For this review, use the dimensioned drawing (mm, ordinates from the lowest corner) and the shaded views. Coordinates: 2 decimals unless noted, no trailing zeros. Loops run counter-clockwise (first coordinate to the right, second up) from the corner with the lowest first, then second, coordinate; pieces in that order, holes last.
1. Take a section at B-B, the plane z = 15. State the section outline as (x, y) points, then the cut area to 3 significant figures.
2. Take a section at C-C, the plane x = 53.5. State the section outline as (y, z) points.
3. Mouldability with a two-part tool opening along Y and no side actions: class the marked faces 1 and 2 as pulls with the +Y half, pulls with the -Y half, needs draft (parallel to the pull), parting line crosses it, or undercut.
4. Take a section at D-D, the plane y = 12. State the section outline as (x, z) points.
5. Take a section at A-A, the plane y = 22.5. State the section outline as (x, z) points, then the cut area to 4 significant figures.
6. Clearance check with flat-ended pins moving along their axes: P1, Ø22.5, axis at x = 80.5, y = 12, coming from the +Z side; P2, Ø11, axis at y = 22.5, z = 14.5, coming from the -X side; P3, Ø5.5, axis at x = 53, z = 13, coming from the -Y side. State where each tip first meets the part, or that it passes through.
7. To check wall thickness, follow probe 1 along Y at (x, z) = (114.7, 2); probe 2 along X at (y, z) = (27, 4.25); probe 3 along X at (y, z) = (42.7, 4). State the ranges of each line that lie inside material, in increasing order.
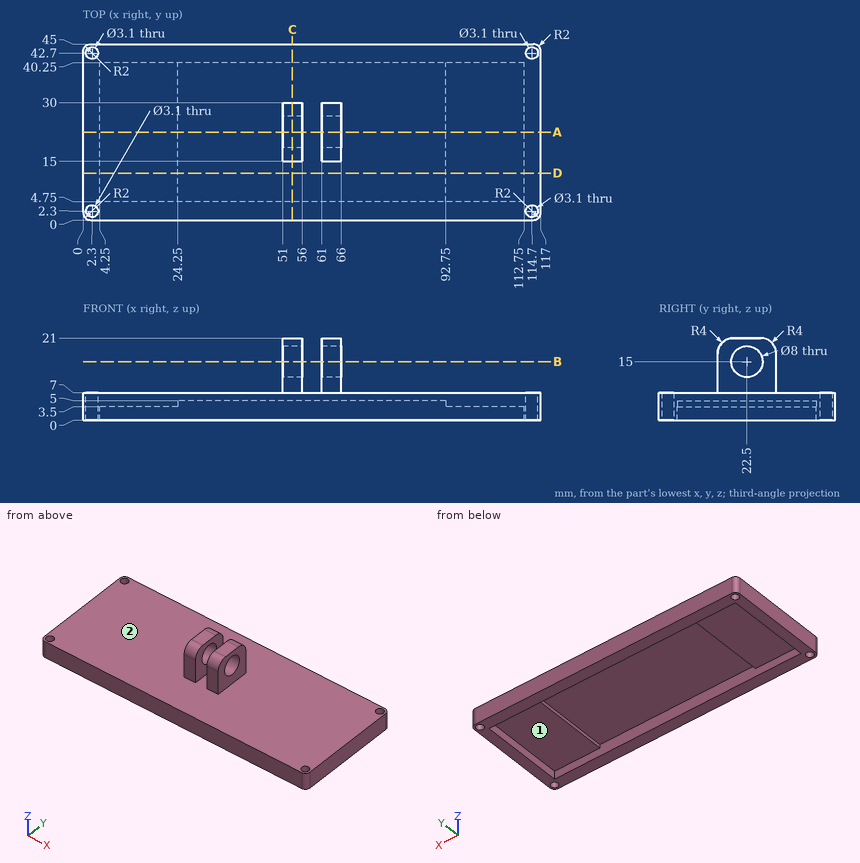
Results list:
1. outline: (51, 15) - (56, 15) - (56, 18.5) - (51, 18.5) - close; (51, 26.5) - (56, 26.5) - (56, 30) - (51, 30) - close; (61, 15) - (66, 15) - (66, 18.5) - (61, 18.5) - close; (61, 26.5) - (66, 26.5) - (66, 30) - (61, 30) - close
1. area: 70.0 mm2
2. outline: (0, 0) - (4.75, 0) - (4.75, 5) - (40.25, 5) - (40.25, 0) - (45, 0) - (45, 7) - (30, 7) - (30, 17) arc R4 ccw to (26, 21) - (19, 21) arc R4 ccw to (15, 17) - (15, 7) - (0, 7) - close; hole circle Ø8 at (22.5, 15)
3. face 1: undercut
3. face 2: needs draft
4. outline: (0, 0) - (4.25, 0) - (4.25, 3.5) - (24.25, 3.5) - (24.25, 5) - (92.75, 5) - (92.75, 3.5) - (112.75, 3.5) - (112.75, 0) - (117, 0) - (117, 7) - (0, 7) - close
5. outline: (0, 0) - (4.25, 0) - (4.25, 3.5) - (24.25, 3.5) - (24.25, 5) - (92.75, 5) - (92.75, 3.5) - (112.75, 3.5) - (112.75, 0) - (117, 0) - (117, 7) - (66, 7) - (66, 11) - (61, 11) - (61, 7) - (56, 7) - (56, 11) - (51, 11) - (51, 7) - (0, 7) - close; (51, 19) - (56, 19) - (56, 21) - (51, 21) - close; (61, 19) - (66, 19) - (66, 21) - (61, 21) - close
5. area: 396.5 mm2
6. P1: stops at z = 7
6. P2: stops at x = 51
6. P3: stops at y = 15
7. probe 1: y = 0 to 0.75, 3.85 to 41.15, 44.25 to 45
7. probe 2: x = 0 to 24.25, 92.75 to 117
7. probe 3: x = 0 to 0.75, 3.85 to 113.15, 116.25 to 117
